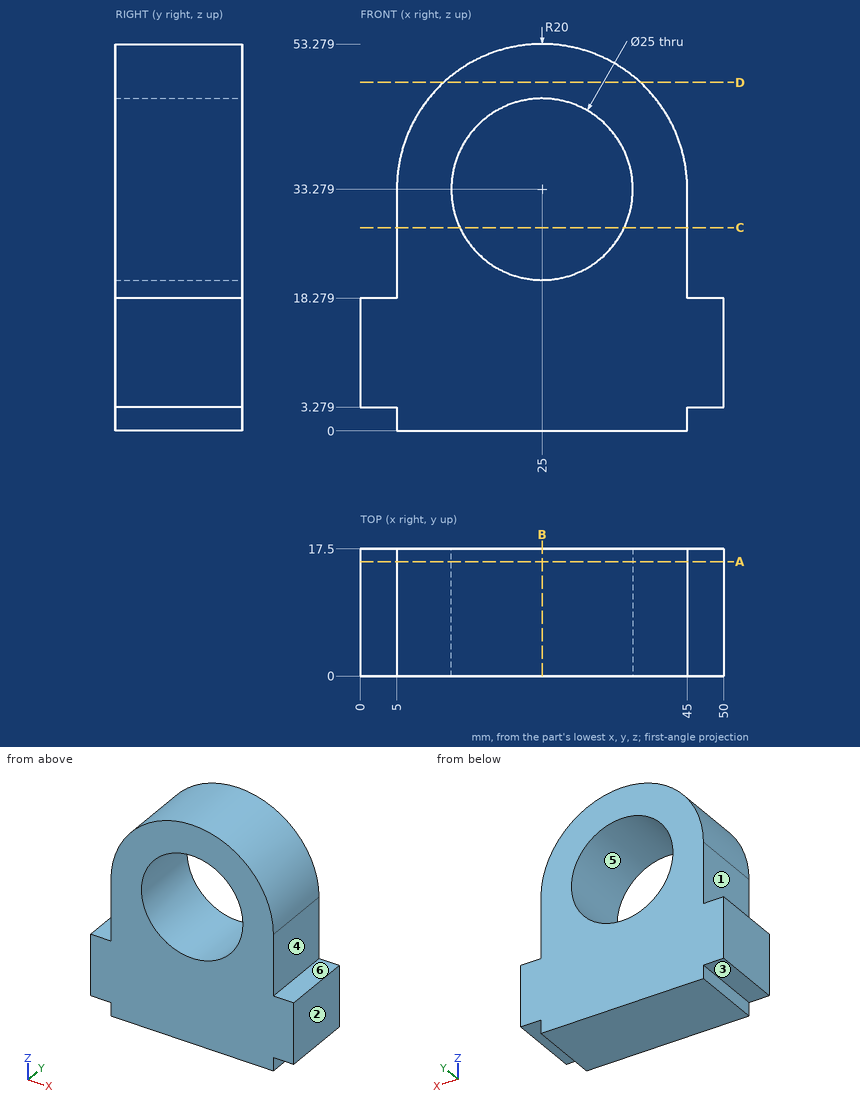
Verification items for this drawing (mm, ordinates from the low corner). A direction names the side the tool comes from. Give positions to 0.01 mm unless a question says otherwise; leave off trailing zeros. Loops run counter-clockwise (first coordinate to the right, second up) from the corner with the lowest first, then second, coordinate; pieces in that order, holes last.
1. Go/stop test with flat-tipped pins: P1, Ø4, axis at x = 27, y = 9, coming from the -Z side; P2, Ø7.5, axis at y = 10, z = 23, coming from the -X side; P3, Ø4, axis at x = 2, y = 6.5, coming from the -Z side; P4, Ø2.5, axis at y = 5.5, z = 1.5, coming from the +X side. Record where each tip stops, or that it passes through.
Derived:
P1: stops at z = 0
P2: stops at x = 5
P3: stops at z = 3.28
P4: stops at x = 45
2. Cross-section at D-D on z = 48. Record the cut outline in (x, y), and give its area (3 significant figures).
Derived:
outline: (11.46, 0) - (38.54, 0) - (38.54, 17.5) - (11.46, 17.5) - close
area: 474 mm2
3. Cross-section at C-C on z = 28. Record the cut outline in (x, y).
Derived:
outline: (5, 0) - (13.67, 0) - (13.67, 17.5) - (5, 17.5) - close; (36.33, 0) - (45, 0) - (45, 17.5) - (36.33, 17.5) - close
4. Cross-section at A-A on y = 15.75. Record the cut outline in (x, z), and give its area (3 significant figures).
Derived:
outline: (0, 3.28) - (5, 3.28) - (5, 0) - (45, 0) - (45, 3.28) - (50, 3.28) - (50, 18.28) - (45, 18.28) - (45, 33.28) arc R20 ccw to (5, 33.28) - (5, 18.28) - (0, 18.28) - close; hole circle Ø25 at (25, 33.28)
area: 1,620 mm2
5. Tool access check on the marked faces 1, 2 and 3. Record the directions out of +Z, -Z, +X, -X, +Y, -Y that give a thin tool (end or side, any length) a straight path to the whole face; none if there is none.
Derived:
face 1: +Z, -X, +Y, -Y
face 2: +Z, -Z, +X, +Y, -Y
face 3: -Z, -X, +Y, -Y
6. Material ranges on probe 1 along Z at (x, y) = (25, 14.25); probe 2 along Z at (x, y) = (2.5, 9.75); probe 3 along X at (y, z) = (2, 38.5), recorded low to high.
Derived:
probe 1: z = 0 to 20.78, 45.78 to 53.28
probe 2: z = 3.28 to 18.28
probe 3: x = 5.69 to 13.64, 36.36 to 44.31
7. Release check for a two-part mould opening along Z. For the marked faces 4, 5 and 6 record: +Z half, -Z half, draft (parallel to the pull), parting line (faces both ways), or undercut.
Derived:
face 4: draft
face 5: undercut
face 6: +Z half
8. Cross-section at B-B on x = 25. Record the cut outline in (y, z).
Derived:
outline: (0, 0) - (17.5, 0) - (17.5, 20.78) - (0, 20.78) - close; (0, 45.78) - (17.5, 45.78) - (17.5, 53.28) - (0, 53.28) - close
